Source: CAD feature listing. Evaluate the final solid. Frame: model axes, mm. A direction names the side the tool comes from. Give positions to 0.01 mm unless a question says otherwise; leave off trailing zeros. Write each loop counter-clockwise with the first axis right and the second up, starting at its lowest first coordinate (ties: lowest second). Pieces come first, ordered by that corner, then holes. Notation, with made-up numbers: (11.25, 58) -> (44.25, 58) arc R27 cw to (44.25, 82) -> close; hole circle Ø11 at (84, 81.5). An arc over 180 degrees is marked (long way). Use a Markdown table: item, result. Add a question column.
```python
from build123d import *

# Parameters (mm, degrees)
SKETCH2_W           = 76.2
SKETCH2_H           = 76.2
SKETCH2_W_2         = 69.85
SKETCH2_H_2         = 69.85
BOSS_EXTRUDE1_DEPTH = 208.2
SKETCH3_R           = 15.875
SKETCH3_R_2         = 7.9375
CUT_EXTRUDE1_DEPTH  = 225.956195736


with BuildPart() as part:
    # Sketch2 → Boss-Extrude1 (new, symmetric)
    with BuildSketch(Plane.XY):
        Rectangle(SKETCH2_W, SKETCH2_H)
        Rectangle(SKETCH2_W_2, SKETCH2_H_2, mode=Mode.SUBTRACT)
    extrude(amount=BOSS_EXTRUDE1_DEPTH, both=True)

    # Sketch3 → Cut-Extrude1 (cut, through all)
    with BuildSketch(Plane.ZY.offset(38.1)):
        with Locations(Location((0, 0, 0), (0, 0, 270))):
            Circle(SKETCH3_R)
        with Locations(Location((-49.4109375, 0, 0), (0, 0, 270))):
            Circle(SKETCH3_R_2)
        with Locations(Location((49.4109375, 0, 0), (0, 0, 270))):
            Circle(SKETCH3_R_2)
    extrude(amount=-CUT_EXTRUDE1_DEPTH, mode=Mode.SUBTRACT)


solid = part.part
```
(1) Access query for faces 1 (the cylindrical face through (-36.535, 3.441, -15.497)), 2 (the flat face through (34.925, -16, 3)). Directions: +Z, -Z, +X, -X, +Y, -Y. A direction counts if a zero-diameter tool reaches every point of the face in a straight line with its end or side. Return the directions, or none.
(2) Cut plane D-D on y = 0. Count the separate pieces of the cut face and the enclosed holes in it, then the cut area to 3 significant figures.
(3) Cut plane A-A on z = 0. Return the cut outline in (x, y) (3 decimals), then the cut area to 3 significant figures.
(4) Material intervals for L1, parallel to Z at x = -36, y = 0 (3 decimals); L2, parallel to Y at x = 2.5, z = 46.5 (3 decimals), sorted ascending.
(5) Mould query, pull axis Z, two halves, no side actions, for faces 3 (the flat face through (-34.925, -16, 3)), 4 (the cylindrical face through (-36.53, 1.72, 41.66)), 5 (the flat face through (-3, -37, -208.2)). Classes: +Z half, -Z half, draft (parallel to the pull), parting line (faces both ways), or undercut.
(6) Cut plane B-B on y = -28. Return the cut outline in (x, z) (3 decimals), then the cut area to 3 significant figures.
(7) First-contact query: pin 1 Ø19 at (y, z) = (0, 0) entering from +X; pin 2 Ø20.5 at (y, z) = (0, 49.41) entering from +X. Flat tips, straight axial feed; report the tip coordinate or a pass-through.
Output:
| question | item | result |
|---|---|---|
| 1 | face 1 | +X, -X |
| 1 | face 2 | +Z, -Z |
| 2 | separate pieces | 8 |
| 2 | enclosed holes | 0 |
| 2 | area | 2,240 mm^2 |
| 3 | outline | (-38.1, -38.1) -> (38.1, -38.1) -> (38.1, -15.875) -> (34.925, -15.875) -> (34.925, -34.925) -> (-34.925, -34.925) -> (-34.925, -15.875) -> (-38.1, -15.875) -> close; (-38.1, 15.875) -> (-34.925, 15.875) -> (-34.925, 34.925) -> (34.925, 34.925) -> (34.925, 15.875) -> (38.1, 15.875) -> (38.1, 38.1) -> (-38.1, 38.1) -> close |
| 3 | area | 726 mm^2 |
| 4 | L1 | -208.2 to -57.348, -41.473 to -15.875, 15.875 to 41.473, 57.348 to 208.2 |
| 4 | L2 | -38.1 to -34.925, 34.925 to 38.1 |
| 5 | face 3 | draft |
| 5 | face 4 | undercut |
| 5 | face 5 | -Z half |
| 6 | outline | (-38.1, -208.2) -> (-34.925, -208.2) -> (-34.925, 208.2) -> (-38.1, 208.2) -> close; (34.925, -208.2) -> (38.1, -208.2) -> (38.1, 208.2) -> (34.925, 208.2) -> close |
| 6 | area | 2,640 mm^2 |
| 7 | pin 1 | through |
| 7 | pin 2 | x = 38.1 |
